Autodesk Inventor part; units mm, degrees
ref_plane "YZ Plane" through (0, 0, 0) normal (1, 0, 0) x (0, 1, 0)
ref_plane "XZ Plane" through (0, 0, 0) normal (0, 1, 0) x (-1, 0, 0)
ref_plane "XY Plane" through (0, 0, 0) normal (0, 0, 1) x (1, 0, 0)
sketch "Sketch1" plane through (0, 0, 0) normal (0, 1, 0) x (-1, 0, 0)
  line L0 (10, 27.8) -> (-10, 27.8)
  line L1 (-10, 27.8) -> (-10, -27.8)
  line L2 (-10, -27.8) -> (10, -27.8)
  line L3 (10, -27.8) -> (10, 27.8)
  line L4 (10, 27.8) -> (-10, -27.8) construction
  line L5 (-10, 27.8) -> (10, -27.8) construction
  point P0 (0, 0)
  dimension "d0" = 55.6
  dimension "d1" = 20
extrude "Plate1" add sketch "Sketch1" along normal blind 3.048
sketch "Sketch2" plane through (10, 0, 27.8) normal (0, 0, -1) x (-1, 0, 0)
  line L0 (20, 3.048) -> (0, 3.048)
  line L1 (0, 3.048) -> (0, 25.4)
  line L2 (0, 25.4) -> (20, 25.4)
  line L3 (20, 25.4) -> (20, 3.048)
edge flange "Flange1" height 25.4 angle 90 thickness 3.048 bend radius 3.048 thickness toward (0, 0, -1) relief tear relief width 3.048 relief depth 1.524 edges at (0, 3.048, 27.8) wall of the first edge with corners at (-10, 3.048, 27.8) (10, 3.048, 27.8) (10, 25.4, 27.8) (-10, 25.4, 27.8)
bend "Bend1"
corner "Corner1"
sketch "Sketch3" plane through (-10, 0, -27.8) normal (0, 0, 1) x (1, 0, 0)
  line L0 (20, 3.048) -> (0, 3.048)
  line L1 (0, 3.048) -> (0, 25.4)
  line L2 (0, 25.4) -> (20, 25.4)
  line L3 (20, 25.4) -> (20, 3.048)
edge flange "Flange2" height 25.4 angle 90 thickness 3.048 bend radius 3.048 thickness toward (0, 0, 1) relief tear relief width 3.048 relief depth 1.524 edges at (0, 3.048, -27.8) wall of the first edge with corners at (10, 3.048, -27.8) (-10, 3.048, -27.8) (-10, 25.4, -27.8) (10, 25.4, -27.8)
bend "Bend2"
corner "Corner2"
equation "\"d2\" = Thickness"
equation "\"d3\" = BendReliefWidth"
equation "\"d4\" = BendReliefDepth"
equation "\"d5\" = MinimumRemnant"
equation "\"d6\" = TransitionRadius"
equation "\"d9\" = BendRadius"
equation "\"d10\" = CornerReliefSize"
equation "\"d11\" = GapSize"
equation "\"d12\" = JacobiRadiusSize"
equation "\"d13\" = BendReliefWidth"
equation "\"d14\" = BendReliefDepth"
equation "\"d15\" = MinimumRemnant"
equation "\"d16\" = TransitionRadius"
equation "\"d19\" = BendRadius"
equation "\"d20\" = CornerReliefSize"
equation "\"d21\" = GapSize"
equation "\"d22\" = JacobiRadiusSize"
equation "\"BendRadius\" = Thickness"
equation "\"BendReliefWidth\" = Thickness"
equation "\"BendReliefDepth\" = 0.5 * Thickness"
equation "\"CornerReliefSize\" = 4 * Thickness"
equation "\"MinimumRemnant\" = 2 * Thickness"
equation "\"TransitionRadius\" = BendRadius"
equation "\"JacobiRadiusSize\" = BendRadius"
equation "\"GapSize\" = Thickness"
properties part number "bracket1"
For this review, take the finished solid that the model builds, in its own axes (mm). A direction names the side the tool comes from. Coordinates: 2 decimals unless noted, no trailing zeros. Order: outer loops, then holes, each group sorted by start corner. A loop starts at its lowest first (then second) coordinate and runs counter-clockwise, first axis right, second up. Notation, with made-up numbers: (-10, 48.25) -> (1, 48.25) arc R38 cw to (1, 86.25) -> close; hole circle Ø6 at (69, 16). An arc over 180 degrees is marked (long way). Use CSV: the item, a comma, the result in double quotes. Start each with the question number.
Item 1: We need section C-C, the plane z = 13.5. Give the boundary of the cut face in (x, y), then the cut area to 3 significant figures.
Item 2: We need section A-A, the plane y = 14. Give the boundary of the cut face in (x, z), then the cut area to 3 significant figures.
Item 3: Insertion check: pin 1 (12 mm diameter, centred on x = 5, z = 13.5, fed in from +Y). The pin has a flat end and moves straight along its axis. Give the tip position at first contact, or say it passes through.
Item 4: Draft analysis for pull direction Z (two halves, no side actions). For faces 1 (the face through (0, 16, -27.8)), 2 (the face through (-0.14, 3.96, -23.88)), 3 (the face through (0, 16, 27.8)), state which applies: pulls with the +Z half, pulls with the -Z half, needs draft (parallel to the pull), parting line crosses it, or undercut.
Item 5: We need section D-D, the plane y = 2.5. Give the boundary of the cut face in (x, z).
Item 6: We need section B-B, the plane x = -1.25. Give the boundary of the cut face in (y, z), then the cut area to 3 significant figures.
Item 7: For faces 4 (the face through (-10, 2, -2)), 5 (the face through (0, 16, -24.752)), list the 3-axis set-ups (+Z, -Z, +X, -X, +Y, -Y) from which the entire face can be reached by the end or side of a thin tool; tool diameter is ignored.
Item 8: Wall thickness on probe 1 along Z at (x, y) = (-5.25, 9); probe 2 along Y at (x, z) = (6.25, -5.5); probe 3 along Z at (x, y) = (-0.5, 5.25): over which ranges is each line inside the solid? List them lowest first.
Derived:
1,outline,"(-10, 0) -> (10, 0) -> (10, 3.05) -> (-10, 3.05) -> close"
1,area,"61.0 mm^2"
2,outline,"(-10, -27.8) -> (10, -27.8) -> (10, -24.75) -> (-10, -24.75) -> close; (-10, 24.75) -> (10, 24.75) -> (10, 27.8) -> (-10, 27.8) -> close"
2,area,"122 mm^2"
3,pin 1,"stops at y = 3.05"
4,face 1,"pulls with the -Z half"
4,face 2,"undercut"
4,face 3,"pulls with the +Z half"
5,outline,"(-10, -26.63) -> (10, -26.63) -> (10, 26.63) -> (-10, 26.63) -> close"
6,outline,"(0, -21.7) arc R6.1 ccw to (6.1, -27.8) -> (25.4, -27.8) -> (25.4, -24.75) -> (6.1, -24.75) arc R3.05 cw to (3.05, -21.7) -> (3.05, 21.7) arc R3.05 cw to (6.1, 24.75) -> (25.4, 24.75) -> (25.4, 27.8) -> (6.1, 27.8) arc R6.1 ccw to (0, 21.7) -> close"
6,area,"294 mm^2"
7,face 4,"+Z, -Z, -X, +Y, -Y"
7,face 5,"+X, -X, +Y"
8,probe 1,"z = -27.8 to -24.75, 24.75 to 27.8"
8,probe 2,"y = 0 to 3.05"
8,probe 3,"z = -27.74 to -24.63, 24.63 to 27.74"
